The listing builds one solid part. Answer for the finished solid, in the listing's coordinates (mm). A direction names the side the tool comes from. Round coordinates to 2 decimals unless told otherwise and drop trailing zeros. Write each loop counter-clockwise with the first axis right and the second up, starting at its lowest first coordinate (ties: lowest second). Pieces come first, ordered by that corner, then holes. Notation, with made-up numbers: (-31.5, -23.5) - (2.5, -23.5) arc R8 ccw to (2.5, -10.5) - close; hole circle Ø1 at (-12.75, 58.5). An arc over 180 degrees is marked (long way). Answer in a Markdown table with one row per item.
from build123d import *

# Parameters (mm, degrees)
SKETCH1_W           = 80
SKETCH1_H           = 50
SKETCH1_R           = 3
BOSS_EXTRUDE1_DEPTH = 5
CUT_EXTRUDE1_DEPTH  = 5
SKETCH4_R           = 1.5
SKETCH4_R_2         = 2
CUT_EXTRUDE2_DEPTH  = 10


with BuildPart() as part:
    # Sketch1 → Boss-Extrude1 (new body)
    with BuildSketch(Plane(origin=(0, 0, 0), x_dir=(1, 0, 0), z_dir=(0, 1, 0))):
        with Locations((40, 25)):
            Rectangle(SKETCH1_W, SKETCH1_H)
        with Locations(Location((65, 10, 0), (0, 0, 270))):
            Circle(SKETCH1_R, mode=Mode.SUBTRACT)
        with Locations(Location((65, 40, 0), (0, 0, 270))):
            Circle(SKETCH1_R, mode=Mode.SUBTRACT)
    extrude(amount=BOSS_EXTRUDE1_DEPTH)

    # Sketch2 → Cut-Extrude1 (cut)
    with BuildSketch(Plane(origin=(0, 5, 0), x_dir=(1, 0, 0), z_dir=(0, 1, 0))):
        with BuildLine():
            Line((37.752664082, 43), (45.752664082, 43))
            ThreePointArc((45.752664082, 43), (48.752664082, 40), (45.752664082, 37))
            Line((45.752664082, 37), (37.752664082, 37))
            ThreePointArc((37.752664082, 37), (34.752664082, 40), (37.752664082, 43))
        make_face()
    extrude(amount=-CUT_EXTRUDE1_DEPTH, mode=Mode.SUBTRACT)

    # Sketch4 → Cut-Extrude2 (cut)
    with BuildSketch(Plane(origin=(0, 5, 0), x_dir=(1, 0, 0), z_dir=(0, 1, 0))):
        with Locations(Location((37.752664082, 24.743683398, 0), (0, 0, 270))):
            Circle(SKETCH4_R)
        with Locations(Location((27.752664082, 24.743683398, 0), (0, 0, 270))):
            Circle(SKETCH4_R)
        with Locations(Location((5, 30, 0), (0, 0, 270))):
            Circle(SKETCH4_R_2)
        with Locations(Location((5, 5, 0), (0, 0, 270))):
            Circle(SKETCH4_R_2)
    extrude(amount=-CUT_EXTRUDE2_DEPTH, mode=Mode.SUBTRACT)


solid = part.part
(1) For a pull along Z with two mould halves and no side action, classify faces 1 (the flat face through (39, 2, -50)), 2 (the flat face through (0, 2, -25)), 3 (the cylindrical face through (34.753, 2.535, -39.934)) as pulls with the +Z half, pulls with the -Z half, needs draft (parallel to the pull), parting line crosses it, or undercut.
Checked values:
| item | result |
|---|---|
| face 1 | pulls with the -Z half |
| face 2 | needs draft |
| face 3 | undercut |
(2) Section D-D (y = 3.7) is taken. Give the vertices of the cut face in (x, z), and give its area (3 significant figures).
Checked values:
| item | result |
|---|---|
| outline | (0, -50) - (80, -50) - (80, 0) - (0, 0) - close; hole circle Ø4 at (5, -30); hole circle Ø4 at (5, -5); hole circle Ø3 at (27.75, -24.74); hole circle Ø3 at (37.75, -24.74); hole (37.75, -43) - (45.75, -43) arc R3 ccw to (45.75, -37) - (37.75, -37) arc R3 ccw to start; hole circle Ø6 at (65, -40); hole circle Ø6 at (65, -10) |
| area | 3,830 mm2 |
(3) A flat-ended cylindrical pin translates along its axis: pin 1 (2.5 mm diameter, centred on x = 27.75, z = -24.74, fed in from +Y). Find the tip coordinate at first contact, or state that the pin passes through.
Checked values:
| item | result |
|---|---|
| pin 1 | passes through |
(4) Section C-C (z = -30) is taken. Give the vertices of the cut face in (x, y), and give its area (3 significant figures).
Checked values:
| item | result |
|---|---|
| outline | (0, 0) - (3, 0) - (3, 5) - (0, 5) - close; (7, 0) - (80, 0) - (80, 5) - (7, 5) - close |
| area | 380 mm2 |
(5) Find the intervals of material crossed by line 1 (X direction, y = 1.7, z = -40); line 2 (Z direction, x = 42, y = 2.6); line 3 (X direction, y = 3, z = -26), in increasing order.
Checked values:
| item | result |
|---|---|
| line 1 | x = 0 to 34.75, 48.75 to 62, 68 to 80 |
| line 2 | z = -50 to -43, -37 to 0 |
| line 3 | x = 0 to 26.93, 28.57 to 36.93, 38.57 to 80 |
(6) Section A-A (x = 65) is taken. Give the vertices of the cut face in (y, z).
Checked values:
| item | result |
|---|---|
| outline | (0, -50) - (5, -50) - (5, -43) - (0, -43) - close; (0, -37) - (5, -37) - (5, -13) - (0, -13) - close; (0, -7) - (5, -7) - (5, 0) - (0, 0) - close |
(7) For faces 4 (the cylindrical face through (48.75, 2.54, -40.07)), 5 (the flat face through (80, 2, -25)), determine the directions among +Z, -Z, +X, -X, +Y, -Y from which every point of the face is accessible in a straight line to the end or side of a thin tool.
Checked values:
| item | result |
|---|---|
| face 4 | +Y, -Y |
| face 5 | +Z, -Z, +X, +Y, -Y |
(8) Section B-B (z = -40) is taken. Give the vertices of the cut face in (x, y), and give its area (3 significant figures).
Checked values:
| item | result |
|---|---|
| outline | (0, 0) - (34.75, 0) - (34.75, 5) - (0, 5) - close; (48.75, 0) - (62, 0) - (62, 5) - (48.75, 5) - close; (68, 0) - (80, 0) - (80, 5) - (68, 5) - close |
| area | 300 mm2 |
